The model under review builds one solid part; all positions refer to its coordinate system, in mm. A direction names the side the tool comes from. Give positions to 0.01 mm unless a question says otherwise; leave off trailing zeros. Order: outer loops, then holes, each group sorted by start corner. A loop starts at its lowest first (then second) coordinate and runs counter-clockwise, first axis right, second up. Notation, with made-up numbers: (48.5, -2.75) - (76.5, -2.75) arc R29 ccw to (76.5, 33.25) - close; hole circle Ø9 at (16.5, 66). An arc over 180 degrees is marked (long way). Put each result on its own line as item: value.
```python
from build123d import *

# Parameters (mm, degrees)
SKETCH1_W           = 95.25
SKETCH1_H           = 292.1
BOSS_EXTRUDE1_DEPTH = 6.35
SKETCH2_W           = 6.35
SKETCH2_H           = 12.7
CUT_EXTRUDE1_DEPTH  = 7.35
LPATTERN1_COUNT     = 12
LPATTERN1_PITCH     = 25.4
SKETCH3_W           = 6.35
SKETCH3_H           = 12.7
CUT_EXTRUDE2_DEPTH  = 7.35
LPATTERN2_COUNT     = 4
LPATTERN2_PITCH     = 25.4
SKETCH4_W           = 12.7
SKETCH4_H           = 6.35
CUT_EXTRUDE3_DEPTH  = 7.35
LPATTERN3_COUNT     = 2
LPATTERN3_PITCH     = 25.4
LPATTERN3_COL_COUNT = 2
LPATTERN3_COL_PITCH = 25.4


with BuildPart() as part:
    # Sketch1 → Boss-Extrude1 (new body)
    with BuildSketch(Plane.XY):
        with Locations((47.625, 146.05)):
            Rectangle(SKETCH1_W, SKETCH1_H)
    extrude(amount=BOSS_EXTRUDE1_DEPTH)

    # Sketch2 → Cut-Extrude1 (cut, through all)
    with BuildSketch(Plane.XY.offset(6.35)):
        with Locations((3.175, 6.35)):
            Rectangle(SKETCH2_W, SKETCH2_H)
        with Locations((92.075, 6.35)):
            Rectangle(SKETCH2_W, SKETCH2_H)
    cut_extrude1 = extrude(amount=-CUT_EXTRUDE1_DEPTH, mode=Mode.SUBTRACT)

    # LPattern1: Cut-Extrude1 ×12
    with Locations(*[(0, i * LPATTERN1_PITCH, 0) for i in range(1, LPATTERN1_COUNT)]):
        add(cut_extrude1, mode=Mode.SUBTRACT)

    # Sketch3 → Cut-Extrude2 (cut, through all)
    with BuildSketch(Plane.XY.offset(6.35)):
        with Locations((85.725, 6.35)):
            Rectangle(SKETCH3_W, SKETCH3_H)
        with Locations((9.525, 6.35)):
            Rectangle(SKETCH3_W, SKETCH3_H)
    cut_extrude2 = extrude(amount=-CUT_EXTRUDE2_DEPTH, mode=Mode.SUBTRACT)

    # LPattern2: Cut-Extrude2 ×4
    with Locations(*[(0, i * LPATTERN2_PITCH, 0) for i in range(1, LPATTERN2_COUNT)]):
        add(cut_extrude2, mode=Mode.SUBTRACT)

    # Sketch4 → Cut-Extrude3 (cut, through all)
    with BuildSketch(Plane.XY.offset(6.35)):
        with Locations((47.625, 142.875)):
            Rectangle(SKETCH4_W, SKETCH4_H)
    cut_extrude3 = extrude(amount=-CUT_EXTRUDE3_DEPTH, mode=Mode.SUBTRACT)

    # LPattern3: Cut-Extrude3 ×2
    with Locations(*[(-i * LPATTERN3_PITCH, 0, 0) for i in range(1, LPATTERN3_COUNT)]):
        add(cut_extrude3, mode=Mode.SUBTRACT)

    # LPattern3 col: Cut-Extrude3 ×2
    with Locations(*[(i * LPATTERN3_COL_PITCH, 0, 0) for i in range(1, LPATTERN3_COL_COUNT)]):
        add(cut_extrude3, mode=Mode.SUBTRACT)


solid = part.part
```
(1) Clearance check with flat-ended pins moving along their axes: pin 1 Ø3 at (x, z) = (88, 4) entering from -Y; pin 2 Ø3 at (y, z) = (233, 3) entering from +X; pin 3 Ø1.9 at (y, z) = (288, 2.5) entering from -X; pin 4 Ø2 at (x, y) = (56.5, 79) entering from -Z. State where each tip first meets the part, or that it passes through.
The answers:
pin 1: y = 12.7
pin 2: x = 88.9
pin 3: x = 6.35
pin 4: z = 0
(2) Take a section at C-C, the plane z = 3.25. Count the separate pieces of the cut face and the enclosed holes in it, then the cut area to 3 significant figures.
The answers:
separate pieces: 1
enclosed holes: 3
area: 25,000 mm^2
(3) Take a section at A-A, the plane x = 44.5. Write out the cut boundary in (y, z).
The answers:
outline: (0, 0) - (139.7, 0) - (139.7, 6.35) - (0, 6.35) - close; (146.05, 0) - (292.1, 0) - (292.1, 6.35) - (146.05, 6.35) - close
(4) For faces 1 (the flat face through (28.575, 143, 3)), 2 (the flat face through (6, 76.2, 3)), 3 (the flat face through (95.25, 171, 3)), 4 (the flat face through (89, 88.9, 3)), 5 (the flat face through (82.55, 6, 3)), list the 3-axis set-ups (+Z, -Z, +X, -X, +Y, -Y) from which the entire face can be reached by the end or side of a thin tool; tool diameter is ignored.
The answers:
face 1: +Z, -Z
face 2: +Z, -Z, -X
face 3: +Z, -Z, +X, +Y, -Y
face 4: +Z, -Z, +X
face 5: +Z, -Z, +X, -Y
(5) Wall thickness on L1, parallel to Y at x = 12, z = 4; L2, parallel to Y at x = 17, z = 5.25; L3, parallel to X at y = 78.5, z = 2.5: over which ranges is each line inside the solid? List them lowest first.
The answers:
L1: 12.7 to 25.4, 38.1 to 50.8, 63.5 to 76.2, 88.9 to 292.1
L2: 0 to 139.7, 146.05 to 292.1
L3: 12.7 to 82.55
(6) Take a section at B-B, the plane x = 9.5. Write out the cut boundary in (y, z).
The answers:
outline: (12.7, 0) - (25.4, 0) - (25.4, 6.35) - (12.7, 6.35) - close; (38.1, 0) - (50.8, 0) - (50.8, 6.35) - (38.1, 6.35) - close; (63.5, 0) - (76.2, 0) - (76.2, 6.35) - (63.5, 6.35) - close; (88.9, 0) - (292.1, 0) - (292.1, 6.35) - (88.9, 6.35) - close
(7) Take a section at D-D, the plane y = 137. Write out the cut boundary in (x, z).
The answers:
outline: (6.35, 0) - (88.9, 0) - (88.9, 6.35) - (6.35, 6.35) - close
